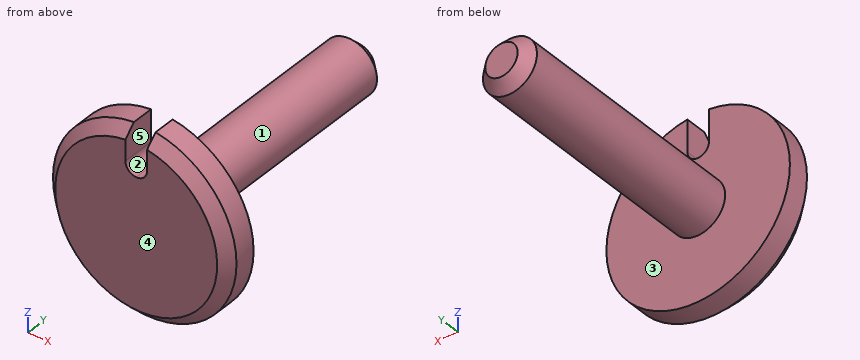
```python
from build123d import *

# Parameters (mm, degrees)
SKETCH1_R           = 2.5
BOSS_EXTRUDE1_DEPTH = 23
CHAMFER1_SIZE       = 1
SKETCH2_R           = 8.5
BOSS_EXTRUDE2_DEPTH = 3
SKETCH3_W           = 2
SKETCH3_H           = 8
CUT_EXTRUDE1_DEPTH  = 3
FILLET1_R           = 1
CHAMFER2_SIZE       = 1


with BuildPart() as part:
    # Sketch1 → Boss-Extrude1 (new body)
    with BuildSketch(Plane(origin=(0, 0, 0), x_dir=(1, 0, 0), z_dir=(0, 1, 0))):
        with Locations(Location((0, 0, 0), (0, 0, 270))):
            Circle(SKETCH1_R)
    extrude(amount=BOSS_EXTRUDE1_DEPTH)

    # Chamfer1
    chamfer1_edges = [part.edges().sort_by_distance(p)[0] for p in [
        (0, 23, -2.5),
    ]]
    chamfer(chamfer1_edges, length=CHAMFER1_SIZE)

    # Sketch2 → Boss-Extrude2 (add)
    with BuildSketch(Plane.XZ):
        with Locations(Location((0, 0, 0), (0, 0, 270))):
            Circle(SKETCH2_R)
    extrude(amount=BOSS_EXTRUDE2_DEPTH)

    # Sketch3 → Cut-Extrude1 (cut)
    with BuildSketch(Plane.XZ.offset(3)):
        with Locations((0, 8.5)):
            Rectangle(SKETCH3_W, SKETCH3_H)
    extrude(amount=-CUT_EXTRUDE1_DEPTH, mode=Mode.SUBTRACT)

    # Fillet1
    fillet1_edges = [part.edges().sort_by_distance(p)[0] for p in [
        (-1, -1.5, 4.5),
        (1, -1.5, 4.5),
    ]]
    fillet(fillet1_edges, radius=FILLET1_R - 0.0001)  # a hair under: the kernel refuses the full size

    # Chamfer2
    chamfer2_edges = [part.edges().sort_by_distance(p)[0] for p in [
        (-8.485230045, -3, -0.500870333),
    ]]
    chamfer(chamfer2_edges, length=CHAMFER2_SIZE)


solid = part.part
```
Geometry check sheet. Reference: the model listing, model coordinates, mm. Face numbers are marked on the shaded views. A direction names the side the tool comes from. Round coordinates to 2 decimals unless told otherwise and drop trailing zeros. Loops run counter-clockwise (first coordinate to the right, second up) from the corner with the lowest first, then second, coordinate; pieces in that order, holes last. Notation, with made-up numbers: (-6.5, 43) - (24.5, 43) arc R18 ccw to (24.5, 62) - close; hole circle Ø3 at (31, 81.25). An arc over 180 degrees is marked (long way). Write each question's results on one line, items separated by ' | '. Start each with the question number.
Q1. Gauge pin test, flat ends, axial feed: P1, Ø10, axis at y = 17.5, z = 5.5, coming from the -X side; P2, Ø2, axis at y = 17, z = 0.5, coming from the +X side; P3, Ø1.5, axis at y = -2, z = 7, coming from the +X side; P4, Ø3, axis at y = 16, z = 5.5, coming from the +X side. Record the tip position at first contact, or that the pin passes through.
Q2. Cross-section at B-B on y = 15. Enter the section's corners in (x, z), and give its area (3 significant figures).
Q3. Thickness scan on line 1 (Y direction, x = 3, z = 3.75); line 2 (Z direction, x = -5.5, y = -1.25); line 3 (Z direction, x = 2.25, y = 10). Record the ranges inside material, lowest first. Write a range as [from, to].
Q4. Release check for a two-part mould opening along X. For the marked faces 1, 2 and 3 record: +X half, -X half, draft (parallel to the pull), parting line (faces both ways), or undercut.
Q5. Cross-section at A-A on z = 0. Enter the section's corners in (x, y), and give its area (3 significant figures).
Q6. Access from +Z, -Z, +X, -X, +Y, -Y to the whole of each face (thin tool, end or side, straight path). Record for the marked faces 4 and 5.
Answers below:
1) P1: stops at x = -2.45 | P2: stops at x = 2.5 | P3: stops at x = 5.76 | P4: passes through
2) outline: circle Ø5 at (0, 0) | area: 19.6 mm²
3) line 1: y = [-3, 0] | line 2: z = [-6.48, 6.48] | line 3: z = [-1.09, 1.09]
4) face 1: parting line | face 2: undercut | face 3: draft
5) outline: (-8.5, -2) - (-7.5, -3) - (7.5, -3) - (8.5, -2) - (8.5, 0) - (2.5, 0) - (2.5, 22) - (1.5, 23) - (-1.5, 23) - (-2.5, 22) - (-2.5, 0) - (-8.5, 0) - close | area: 164 mm²
6) face 4: +Z, -Z, +X, -X, -Y | face 5: +Z, +Y, -Y
